CAD build for the part. Positions are in the model's coordinates, mm. A direction names the side the tool comes from. Give positions to 0.01 mm unless a question says otherwise; leave off trailing zeros. Order: outer loops, then holes, each group sorted by start corner. A loop starts at its lowest first (then second) coordinate and runs counter-clockwise, first axis right, second up. Notation, with made-up numbers: (-27.5, 17) -> (29.5, 17) arc R27 ccw to (29.5, 49) -> close; hole circle Ø9 at (-18, 62). An arc over 180 degrees is marked (long way). Use one line per item in the form item = value. Start each with the question number.
1) Tool access for faces 1 (the face through (76.2, -45, -230)), 2 (the face through (-1, -44.45, -225)): list every direction of +Z, -Z, +X, -X, +Y, -Y with a clear straight run to the whole face (end or side of a thin tool).
2) Cut at A-A, the plane z = -268.5. Give the cut face in (x, y).
3) Probe line 1 (Y direction, x = -22, z = -15); line 2 (Y direction, x = -32, z = -479); line 3 (Z direction, x = -16.5, y = 21). List the from-to ranges inside material, lowest first.
4) Cut at C-C, the plane x = 27.5. Give the cut face in (y, z).
5) Cut at B-B, the plane y = 0. Give the cut face in (x, z), and give its area (3 significant figures).
6) Drop flat-ended pins along their axis: P1, Ø2, axis at x = -48, y = 29.5, coming from the +Z side; P2, Ø10, axis at x = 24.5, y = -11, coming from the -Z side; P3, Ø2, axis at x = -14, y = -22, coming from the -Z side. Give the stop position or say it passes through.
7) Mould opens along Z. For faces 3 (the face through (-76.2, 45, -230)), 4 (the face through (-1.07, -1.03, 46.98)), 5 (the face through (1.07, 0.98, -501.64)), 6 (the face through (-1.07, 1.03, -504.18)) say: pulls with the +Z half, pulls with the -Z half, needs draft (parallel to the pull), parting line crosses it, or undercut.
from build123d import *

# Parameters (mm, degrees)
SKETCH1_W = 152.4
SKETCH1_H = 2.54


with BuildPart() as part:
    # Sweep1: sweep along a path in Sketch2
    with BuildLine(Plane(origin=(0, 0, 0), x_dir=(0, 0, -1), z_dir=(1, 0, 0))) as sweep1_path:
        Line((0, 45.72), (457.2, 45.72))
        ThreePointArc((457.2, 45.72), (502.92, 0), (457.2, -45.72))
        Line((457.2, -45.72), (0, -45.72))
        ThreePointArc((0, -45.72), (-45.72, 0), (0, 45.72))
    # Sketch1 → Sweep1 (sweep)
    with BuildSketch(Plane.XY):
        with Locations((0, 45.72)):
            Rectangle(SKETCH1_W, SKETCH1_H)
    sweep(path=sweep1_path.line)


solid = part.part
Result:
q1.face_1 = +Z, -Z, +X, +Y, -Y
q1.face_2 = +X, -X
q2.outline = (-76.2, -46.99) -> (76.2, -46.99) -> (76.2, -44.45) -> (-76.2, -44.45) -> close; (-76.2, 44.45) -> (76.2, 44.45) -> (76.2, 46.99) -> (-76.2, 46.99) -> close
q3.line_1 = -46.99 to -44.45, 44.45 to 46.99
q3.line_2 = -41.63 to -38.74, 38.74 to 41.63
q3.line_3 = -499.24 to -496.38, 39.18 to 42.04
q4.outline = (-46.99, -457.2) arc R46.99 ccw to (46.99, -457.2) -> (46.99, 0) arc R46.99 ccw to (-46.99, 0) -> close; hole (-44.45, -457.2) arc R44.45 ccw to (44.45, -457.2) -> (44.45, 0) arc R44.45 ccw to (-44.45, 0) -> close
q5.outline = (-76.2, -504.19) -> (76.2, -504.19) -> (76.2, -501.65) -> (-76.2, -501.65) -> close; (-76.2, 44.45) -> (76.2, 44.45) -> (76.2, 46.99) -> (-76.2, 46.99) -> close
q5.area = 774 mm²
q6.P1 = 37.36
q6.P2 = -503.81
q6.P3 = -499.24
q7.face_3 = needs draft
q7.face_4 = pulls with the +Z half
q7.face_5 = undercut
q7.face_6 = pulls with the -Z half
